```python
from build123d import *

# Parameters (mm, degrees)
SKETCH1_W                = 33
SKETCH1_H                = 33
BOSS_EXTRUDE1_DEPTH      = 33
SKETCH2_W                = 21
SKETCH2_H                = 21
CUT_EXTRUDE1_DEPTH       = 58.15767665
SKETCH3_W                = 21
SKETCH3_H                = 21
CUT_EXTRUDE2_DEPTH       = 58.15767665
SKETCH4_W                = 21
SKETCH4_H                = 21
CUT_EXTRUDE3_DEPTH       = 58.15767665
SKETCH5_R                = 3.05
CUT_EXTRUDE4_DEPTH       = 58.15767665
SKETCH6_R                = 3.05
CUT_EXTRUDE5_DEPTH       = 58.15767665
SKETCH7_R                = 3.05
CUT_EXTRUDE6_DEPTH       = 58.15767665
BOSS_EXTRUDE7_DEPTH      = 12
CUT_EXTRUDE7_REACH       = 66.831
SKETCH14_R               = 3.05
FILLET1_R                = 6
CHAMFER1_START           = -1
CHAMFER1_OUTLINE_W       = 16
CHAMFER1_OUTLINE_H       = 18
CHAMFER1_DEPTH           = 6.773502692
BOSS_EXTRUDE3_DEPTH      = 8
BOSS_EXTRUDE3_DEPTH_BACK = 10
SKETCH9_W                = 18
SKETCH9_H                = 18
CHAMFER2_SIZE            = 6
FILLET2_R                = 1.25
SKETCH10_R               = 6
BOSS_EXTRUDE4_DEPTH      = 10
SKETCH11_R               = 6
BOSS_EXTRUDE5_DEPTH      = 10
SKETCH12_R               = 6
BOSS_EXTRUDE6_DEPTH      = 10
FILLET3_R                = 2
FILLET4_R                = 2.5


with BuildPart() as part:
    # Sketch1 → Boss-Extrude1 (new body)
    with BuildSketch(Plane(origin=(0, 0, 0), x_dir=(1, 0, 0), z_dir=(0, 1, 0))):
        with Locations((16.5, -16.5)):
            Rectangle(SKETCH1_W, SKETCH1_H)
    extrude(amount=BOSS_EXTRUDE1_DEPTH)

    # Sketch2 → Cut-Extrude1 (cut, through all)
    with BuildSketch(Plane.XY.offset(33)):
        with Locations((22.5, 22.5)):
            Rectangle(SKETCH2_W, SKETCH2_H)
    extrude(amount=-CUT_EXTRUDE1_DEPTH, mode=Mode.SUBTRACT)

    # Sketch3 → Cut-Extrude2 (cut, through all)
    with BuildSketch(Plane.XZ):
        with Locations((22.5, 22.5)):
            Rectangle(SKETCH3_W, SKETCH3_H)
    extrude(amount=-CUT_EXTRUDE2_DEPTH, mode=Mode.SUBTRACT)

    # Sketch4 → Cut-Extrude3 (cut, through all)
    with BuildSketch(Plane.ZY):
        with Locations((22.5, 22.5)):
            Rectangle(SKETCH4_W, SKETCH4_H)
    extrude(amount=-CUT_EXTRUDE3_DEPTH, mode=Mode.SUBTRACT)

    # Sketch5 → Cut-Extrude4 (cut, through all)
    with BuildSketch(Plane.ZY):
        with Locations((27, 6)):
            Circle(SKETCH5_R)
        with Locations((6, 18)):
            Circle(SKETCH5_R)
    extrude(amount=-CUT_EXTRUDE4_DEPTH, mode=Mode.SUBTRACT)

    # Sketch6 → Cut-Extrude5 (cut, through all)
    with BuildSketch(Plane.XZ):
        with Locations(Location((6, 18, 0), (0, 0, 270))):
            Circle(SKETCH6_R)
        with Locations(Location((27, 6, 0), (0, 0, 270))):
            Circle(SKETCH6_R)
    extrude(amount=-CUT_EXTRUDE5_DEPTH, mode=Mode.SUBTRACT)

    # Sketch7 → Cut-Extrude6 (cut, through all)
    with BuildSketch(Plane(origin=(0, 0, 0), x_dir=(-1, 0, 0), z_dir=(0, 0, -1))):
        with Locations((-18, 6)):
            Circle(SKETCH7_R)
        with Locations((-6, 27)):
            Circle(SKETCH7_R)
    extrude(amount=-CUT_EXTRUDE6_DEPTH, mode=Mode.SUBTRACT)

    # Sketch13 → Boss-Extrude7 (add)
    with BuildSketch(Plane(origin=(0, 33, 0), x_dir=(1, 0, 0), z_dir=(0, 1, 0))):
        Polygon((24, 0), (24, -12), (12, -12), (12, -33), (0, -33), (0, 0), align=None)
    extrude(amount=BOSS_EXTRUDE7_DEPTH)

    # Sketch14 → Cut-Extrude7 (cut, up to next)
    with BuildSketch(Plane(origin=(0, 45, 0), x_dir=(1, 0, 0), z_dir=(0, 1, 0)), mode=Mode.PRIVATE) as cut_extrude7_sk1:
        with Locations(Location((18, -6, 0), (0, 0, 270))):
            Circle(SKETCH14_R)
    cut_extrude7_tool1 = extrude(cut_extrude7_sk1.sketch, amount=-CUT_EXTRUDE7_REACH, mode=Mode.PRIVATE) & part.part
    # Sketch14 → Cut-Extrude7 (cut, up to next)
    with BuildSketch(Plane(origin=(0, 45, 0), x_dir=(1, 0, 0), z_dir=(0, 1, 0)), mode=Mode.PRIVATE) as cut_extrude7_sk2:
        with Locations(Location((6, -27, 0), (0, 0, 270))):
            Circle(SKETCH14_R)
    cut_extrude7_tool2 = extrude(cut_extrude7_sk2.sketch, amount=-CUT_EXTRUDE7_REACH, mode=Mode.PRIVATE) & part.part
    add(cut_extrude7_tool1.solids().sort_by_distance((18, 45, 6))[0], mode=Mode.SUBTRACT)
    add(cut_extrude7_tool2.solids().sort_by_distance((6, 45, 27))[0], mode=Mode.SUBTRACT)

    # Fillet1
    fillet1_edges = [part.edges().sort_by_distance(p)[0] for p in [
        (6, 12, 33),
        (6, 0, 33),
        (33, 6, 0),
        (33, 6, 12),
        (24, 39, 0),
        (24, 39, 12),
        (0, 39, 33),
        (12, 39, 33),
    ]]
    fillet(fillet1_edges, radius=FILLET1_R - 0.0001)  # a hair under: the kernel refuses the full size

    # Chamfer1: read off the stored shape, not the designer's step
    # Chamfer1 outline → Chamfer1 (cut)
    with BuildSketch(Plane(origin=(0, 0, 0), x_dir=(0.8164965809277258, -0.40824829046386313, -0.40824829046386313), z_dir=(0.5773502691896258, 0.5773502691896258, 0.5773502691896258)).offset(CHAMFER1_START)):
        with Locations((2, 0)):
            Rectangle(CHAMFER1_OUTLINE_W, CHAMFER1_OUTLINE_H)
    extrude(amount=CHAMFER1_DEPTH, mode=Mode.SUBTRACT)

    # Sketch9 → Boss-Extrude3 (add, two sides: drawn at the far end of the back side and taken through both)
    with BuildSketch(Plane(origin=(0, 0, 0), x_dir=(1, 0, 0), z_dir=(0, 1, 0)).offset(-BOSS_EXTRUDE3_DEPTH_BACK)):
        with Locations((-1, 1)):
            Rectangle(SKETCH9_W, SKETCH9_H)
    extrude(amount=BOSS_EXTRUDE3_DEPTH + BOSS_EXTRUDE3_DEPTH_BACK)

    # Chamfer2
    chamfer2_edges = [part.edges().sort_by_distance(p)[0] for p in [
        (8, -5, 8),
        (8, 8, -5),
        (-5, 8, 8),
    ]]
    chamfer(chamfer2_edges, length=CHAMFER2_SIZE)

    # Fillet2
    # the kernel refuses this fillet: 1.25 mm, written as the material it adds along each edge
    with BuildSketch(Plane(origin=(-4.268829387, 8, 6.268829387), x_dir=(-0.408248290463863, 0.816496580927726, -0.408248290463863), z_dir=(0.7071067811865476, 0, -0.7071067811865476))) as fillet2_piece_1_section:
        with BuildLine():
            CenterArc((FILLET2_R * 1.93185165258, -FILLET2_R), FILLET2_R, 90, 125.264389683)
            Line((FILLET2_R * 1.11535507165, -FILLET2_R * 1.57735026919), (0, 0))
            Line((0, 0), (FILLET2_R * 1.93185165258, 0))
        make_face()
    fillet2_piece_1 = extrude(amount=14.902499954, mode=Mode.PRIVATE)
    fillet2_piece_1 = split(fillet2_piece_1, bisect_by=Plane(origin=(-1.134414693, 11.134414693, 6.268829387), z_dir=(-0.7071067811865476, -0.7071067811865476, 0)), keep=Keep.TOP, mode=Mode.PRIVATE)
    fillet2_piece_1 = split(fillet2_piece_1, bisect_by=Plane(origin=(-4.268829387, 5.865585306, 4.134414694), z_dir=(0, -0.7071067811865476, -0.7071067811865476)), keep=Keep.TOP, mode=Mode.PRIVATE)
    add(fillet2_piece_1)
    with BuildSketch(Plane(origin=(-4.268829387, 6.268829387, 8), x_dir=(-0.4082482904638628, -0.4082482904638628, 0.8164965809277263), z_dir=(0.7071067811865476, -0.7071067811865476, 0))) as fillet2_piece_2_section:
        with BuildLine():
            CenterArc((FILLET2_R * 1.93185165258, FILLET2_R), FILLET2_R, 144.735610317, 125.264389683)
            Line((FILLET2_R * 1.11535507165, FILLET2_R * 1.57735026919), (0, 0))
            Line((0, 0), (FILLET2_R * 1.93185165258, 0))
        make_face()
    fillet2_piece_2 = extrude(amount=14.902499954, mode=Mode.PRIVATE)
    fillet2_piece_2 = split(fillet2_piece_2, bisect_by=Plane(origin=(-4.268829387, 4.134414694, 5.865585306), z_dir=(0, -0.7071067811865476, -0.7071067811865476)), keep=Keep.TOP, mode=Mode.PRIVATE)
    fillet2_piece_2 = split(fillet2_piece_2, bisect_by=Plane(origin=(-1.134414693, 6.268829387, 11.134414693), z_dir=(-0.7071067811865476, 0, -0.7071067811865475)), keep=Keep.TOP, mode=Mode.PRIVATE)
    add(fillet2_piece_2)
    with BuildSketch(Plane(origin=(8, -4.268829387, 6.268829387), x_dir=(0.8164965809277257, -0.40824829046386313, -0.4082482904638633), z_dir=(0, 0.7071067811865476, -0.7071067811865475))) as fillet2_piece_3_section:
        with BuildLine():
            CenterArc((FILLET2_R * 1.93185165258, FILLET2_R), FILLET2_R, 144.735610317, 125.264389683)
            Line((FILLET2_R * 1.11535507165, FILLET2_R * 1.57735026919), (0, 0))
            Line((0, 0), (FILLET2_R * 1.93185165258, 0))
        make_face()
    fillet2_piece_3 = extrude(amount=14.902499954, mode=Mode.PRIVATE)
    fillet2_piece_3 = split(fillet2_piece_3, bisect_by=Plane(origin=(11.134414693, -1.134414693, 6.268829387), z_dir=(-0.7071067811865476, -0.7071067811865476, 0)), keep=Keep.TOP, mode=Mode.PRIVATE)
    fillet2_piece_3 = split(fillet2_piece_3, bisect_by=Plane(origin=(5.865585306, -4.268829387, 4.134414694), z_dir=(-0.7071067811865476, 0, -0.7071067811865475)), keep=Keep.TOP, mode=Mode.PRIVATE)
    add(fillet2_piece_3)

    # Sketch10 → Boss-Extrude4 (add)
    with BuildSketch(Plane.XZ.offset(10)):
        with Locations(Location((-1, -1, 0), (0, 0, 270))):
            Circle(SKETCH10_R)
    extrude(amount=BOSS_EXTRUDE4_DEPTH)

    # Sketch11 → Boss-Extrude5 (add)
    with BuildSketch(Plane.ZY.offset(10)):
        with Locations((-1, -1)):
            Circle(SKETCH11_R)
    extrude(amount=BOSS_EXTRUDE5_DEPTH)

    # Sketch12 → Boss-Extrude6 (add)
    with BuildSketch(Plane(origin=(0, 0, -10), x_dir=(-1, 0, 0), z_dir=(0, 0, -1))):
        with Locations((1, -1)):
            Circle(SKETCH12_R)
    extrude(amount=BOSS_EXTRUDE6_DEPTH)

    # Fillet3
    fillet3_edges = [part.edges().sort_by_distance(p)[0] for p in [
        (8, -4, -10),
        (-4, -10, 8),
        (-10, 8, -4),
        (-10, -1, -10),
        (-4, 8, -10),
        (-10, -4, 8),
        (-10, -10, -1),
        (-1, -10, -10),
        (8, -10, -4),
        (5, -10, 5),
        (5, 5, -10),
        (-10, 5, 5),
    ]]
    fillet(fillet3_edges, radius=FILLET3_R)

    # Fillet4
    fillet4_edges = [part.edges().sort_by_distance(p)[0] for p in [
        (-1, -20, 5),
        (-20, -1, -7),
        (5, -1, -20),
    ]]
    fillet(fillet4_edges, radius=FILLET4_R)


solid = part.part
```
Can you work these out from the model? Positions are in its coordinate system, mm. A direction names the side the tool comes from. Coordinates: 2 decimals unless noted, no trailing zeros. Order: outer loops, then holes, each group sorted by start corner. A loop starts at its lowest first (then second) coordinate and runs counter-clockwise, first axis right, second up.
1. I need wall thicknesses on line 1 (Y direction, x = 6, z = 23); line 2 (Y direction, x = 8.5, z = 27). Which ranges of each line are inside material? Lowest first, please.
2. If we section it at C-C (x = 19): Please give me the cut outline in (y, z), then the cut area to 3 significant figures.
3. If we section it at D-D (y = 25): Please give me the cut outline in (x, z), then the cut area to 3 significant figures.
4. If we section it at B-B (z = 18): Please give me the cut outline in (x, y).
5. Thinking about a two-plate mould opening in X: for faces 1 (the face through (-0.25, -0.18, 8.21)), 2 (the face through (20.57, 39.08, 7.64)), 3 (the face through (-13.698, -6.857, -2.301)), which applies, +X half, -X half, draft (parallel to the pull), parting line (faces both ways), or undercut?
6. If we section it at A-A (y = 35.5): Give the number of separate pieces and of enclosed holes in the cut face, then the cut area to 3 significant figures.
7. I'm going to push flat-ended pins straight in: pin 1 (13.5 mm diameter, centred on x = 18, z = 7.5, fed in from -Y); pin 2 (16.5 mm diameter, centred on y = 32, z = 16.5, fed in from -X); pin 3 (1 mm diameter, centred on x = -14.5, y = 6.5, fed in from +Z); pin 4 (8 mm diameter, centred on x = 7.5, y = 30.5, fed in from -Z). Where does each tip first touch, or does it pass through?
8. For faces 4 (the face through (13, 0, 10)), 5 (the face through (10.289, 39.084, 31.196)), 6 (the face through (8.21, -0.25, -0.18)), 7 (the face through (4.6, 12, 21.1)), 8 (the face through (5, 5, -4)), which set-ups out of +Z, -Z, +X, -X, +Y, -Y let a thin tool reach every point of the face, with its end or its side?
Entries:
1. line 1: y = 0 to 12, 33 to 45
1. line 2: y = 0 to 2.95, 9.05 to 12
2. outline: (0, 0) - (3.12, 0) - (3.12, 12) - (0, 12) - close; (8.88, 0) - (12, 0) - (12, 12) - (8.88, 12) - close; (33, 0.08) - (45, 0.08) - (45, 3.12) - (33, 3.12) - close; (33, 8.88) - (45, 8.88) - (45, 11.92) - (33, 11.92) - close
2. area: 148 mm2
3. outline: (0, 0) - (3.7, 0) - (3.7, 12) - (0, 12) - close; (8.3, 0) - (12, 0) - (12, 12) - (8.3, 12) - close
3. area: 88.7 mm2
4. outline: (0, 0) - (2.95, 0) - (2.95, 12) - (0, 12) - close; (0, 33) - (12, 33) - (12, 45) - (0, 45) - close; (9.05, 0) - (12, 0) - (12, 12) - (9.05, 12) - close
5. face 1: -X half
5. face 2: undercut
5. face 3: draft
6. separate pieces: 1
6. enclosed holes: 2
6. area: 451 mm2
7. pin 1: stops at y = 0
7. pin 2: stops at x = 0
7. pin 3: passes through
7. pin 4: stops at z = 0
8. face 4: +Z, +X, -Y
8. face 5: +Z, +X, +Y
8. face 6: -Z, -Y
8. face 7: +Z, +X, -X
8. face 8: -Z, +X, +Y
